Job drawing, mm, ordinate dimensions from the low corner. One solid piece. A direction names the side the tool comes from. Round coordinates to 2 decimals unless told otherwise and drop trailing zeros. Write each loop counter-clockwise with the first axis right and the second up, starting at its lowest first coordinate (ties: lowest second). Pieces come first, ordered by that corner, then holes.
1) Which spindle directions (+Z, -Z, +X, -X, +Y, -Y) get a long thin tool onto all of the face, cutting with end or side? Do the marked faces 1, 2 and 3. Say none if no direction does.
2) Saw through at A-A (y = 32). Write the cut outline in (x, z), plus the area to 3 significant figures.
3) Saw through at D-D (x = 44.5). Write the cut outline in (y, z).
4) Wall check: probe 1 along Z at (x, y) = (55, 3.75); probe 2 along X at (y, z) = (25, 21); probe 3 along X at (y, z) = (4.5, 25). Give the ranges that are in metal, low to high.
5) Saw through at B-B (z = 25). Write the cut outline in (x, y).
6) Pull direction Z, two halves, no side cores. Call the marked faces 4, 5 and 6: +Z half, -Z half, draft (parallel to the pull), parting line (faces both ways), or undercut.
7) Flat gauge pins, fed straight in: pin 1 (16 mm diameter, centred on x = 55, z = 25, fed in from -Y); pin 2 (10 mm diameter, centred on x = 43, y = 34.5, fed in from +Z); pin 3 (8 mm diameter, centred on y = 27.5, z = 15, fed in from +X); pin 4 (12 mm diameter, centred on x = 15.5, y = 28, fed in from +Z). Where does each tip first touch, or does it go through?
8) Saw through at C-C (x = 54.5). Write the cut outline in (y, z), plus the area to 3 significant figures.
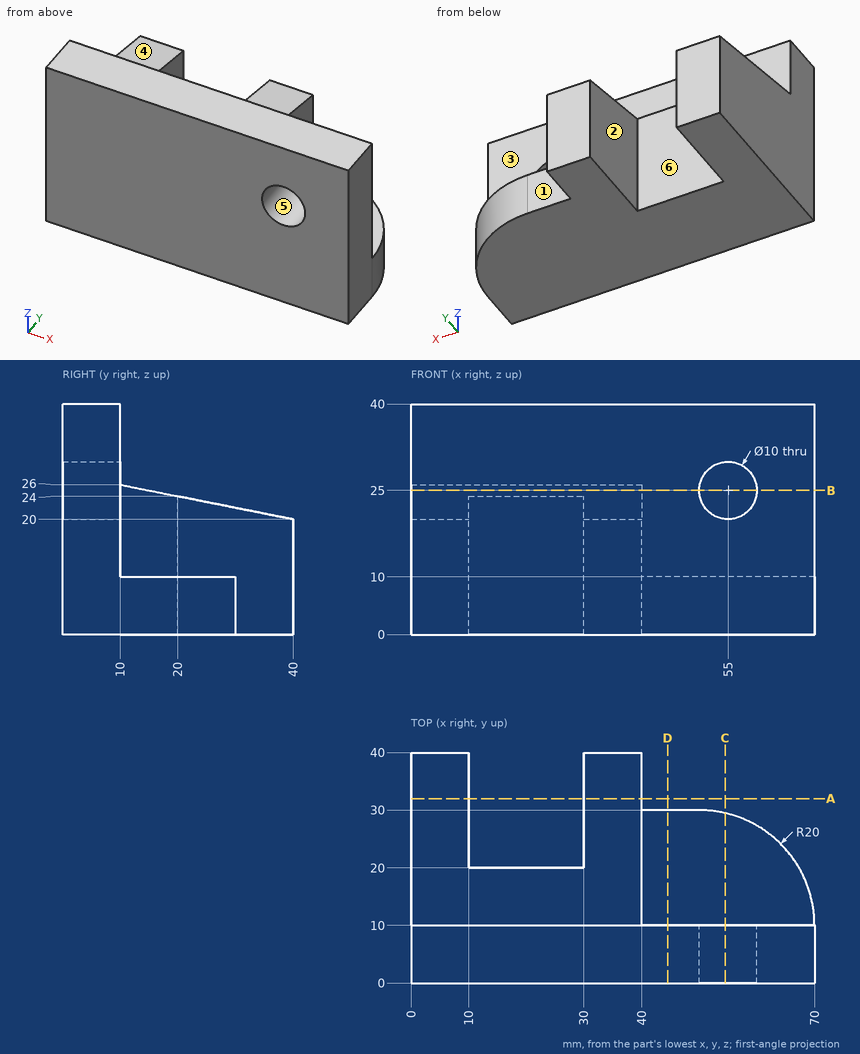
Evaluation:
1. face 1: +Z, -Z, +X, +Y
1. face 2: +Z, -Z, +Y
1. face 3: +Z, +X, +Y
2. outline: (0, 0) - (10, 0) - (10, 21.6) - (0, 21.6) - close; (30, 0) - (40, 0) - (40, 21.6) - (30, 21.6) - close
2. area: 432 mm2
3. outline: (0, 0) - (30, 0) - (30, 10) - (10, 10) - (10, 40) - (0, 40) - close
4. probe 1: z = 0 to 20, 30 to 40
4. probe 2: x = 0 to 10, 30 to 40
4. probe 3: x = 0 to 50, 60 to 70
5. outline: (0, 0) - (50, 0) - (50, 10) - (40, 10) - (40, 15) - (0, 15) - close; (60, 0) - (70, 0) - (70, 10) - (60, 10) - close
6. face 4: +Z half
6. face 5: undercut
6. face 6: draft
7. pin 1: stops at y = 0
7. pin 2: stops at z = 21.9
7. pin 3: stops at x = 40
7. pin 4: stops at z = 22.88
8. outline: (0, 0) - (29.49, 0) - (29.49, 10) - (10, 10) - (10, 20.03) - (0, 20.03) - close; (0, 29.97) - (10, 29.97) - (10, 40) - (0, 40) - close
8. area: 495 mm2
